The listing builds one solid part. Answer for the finished solid, in the listing's coordinates (mm). Face numbers are marked on the shaded views. A direction names the side the tool comes from. Give positions to 0.01 mm unless a question says otherwise; leave off trailing zeros. Write each loop counter-clockwise with the first axis right and the second up, starting at its lowest first coordinate (ties: lowest second). Pieces come first, ordered by that corner, then holes. Notation, with made-up numbers: (64, 22) - (109, 22) arc R14 cw to (109, 41) - close; hole circle Ø1 at (68.5, 16.5). An arc over 180 degrees is marked (long way). Answer as CSV lines item,"result". Start each with the question number.
(1) Find section D-D (x = 5.5). Write down the section's boundary in (y, z), then the cut area to 3 significant figures.
(2) Find section C-C (x = 26). Write down the section's boundary in (y, z).
(3) For a pull along Y with two mould halves and no side action, classify the marked faces 1, 2 and 3 as pulls with the +Y half, pulls with the -Y half, needs draft (parallel to the pull), parting line crosses it, or undercut.
(4) Find section B-B (z = 1). Write down the section's boundary in (x, y).
(5) Find section A-A (y = -3.5). Write down the section's boundary in (x, z), then the cut area to 4 significant figures.
(6) Each of these flat-tipped pins is pushed along its axis until it touches: pin 1 Ø5 at (x, y) = (31, 13) entering from +Z; pin 2 Ø7.5 at (y, z) = (12.5, 0) entering from +X; pin 3 Ø5 at (y, z) = (28.5, 0) entering from -X; pin 4 Ø1.6 at (x, z) = (6.5, 8.5) entering from -Y. Where does it stop, or does it pass through?
(7) Straight lines are drawn through the part: probe 1 along Y at (x, z) = (12.5, 0); probe 2 along X at (y, z) = (12.5, -6.5); probe 3 along Y at (x, z) = (7, 0). For each, find the intervals that lie inside material, in ascending order.
(8) For the marked faces 4, 5, 6, 7 and 8, determine the directions among +Z, -Z, +X, -X, +Y, -Y from which every point of the face is accessible in a straight line to the end or side of a thin tool.
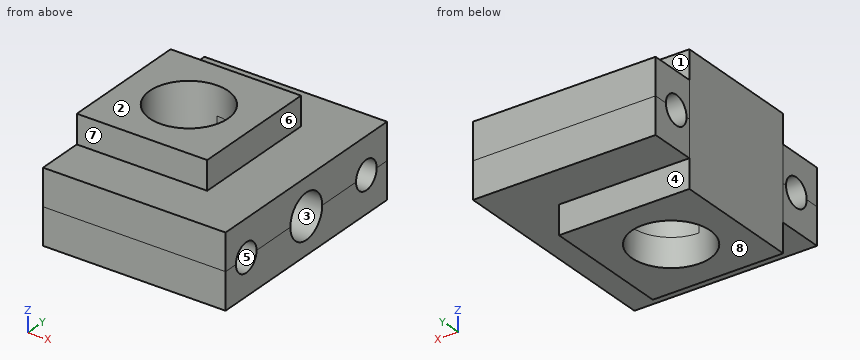
from build123d import *

# Parameters (mm, degrees)
F0_W          = 25
F0_H          = 25
F0_R          = 7.5
F1_DEPTH      = 12.5
F1_DEPTH_BACK = 12.5
F2_W          = 12.5
F2_H          = 9
F3_DEPTH      = 7
F3_DEPTH_BACK = 7
F6_DEPTH      = 10
F5_R          = 2.75
F7_DEPTH      = 35.1


with BuildPart() as f1:
    # F0 (on Top) → F1 (new body, two sides)
    with BuildSketch(Plane.XY) as f1_sk:
        with Locations((12.5, 12.5)):
            Rectangle(F0_W, F0_H)
        with Locations((12.5, 12.5)):
            Circle(F0_R, mode=Mode.SUBTRACT)
    extrude(amount=F1_DEPTH)
    extrude(f1_sk.sketch, amount=-F1_DEPTH_BACK)

    # F2 (on Top) → F3 (join, two sides)
    with BuildSketch(Plane.XY) as f3_sk:
        with BuildLine():
            Line((12.5, 34), (12.5, 25))
            Line((12.5, 25), (12.5, 20))
            ThreePointArc((12.5, 20), (17.803301, 17.803301), (20, 12.5))
            ThreePointArc((20, 12.5), (17.803301, 7.196699), (12.5, 5))
            Line((12.5, 5), (12.5, 0))
            Line((12.5, 0), (12.5, -9))
            Line((12.5, -9), (35, -9))
            Line((35, -9), (35, 34))
            Line((35, 34), (12.5, 34))
        make_face()
        with Locations((6.25, 29.5)):
            Rectangle(F2_W, F2_H)
        with Locations((6.25, -4.5)):
            Rectangle(F2_W, F2_H)
    extrude(amount=F3_DEPTH)
    extrude(f3_sk.sketch, amount=-F3_DEPTH_BACK)

    # F4 (on face) → F6 (cut)
    with BuildSketch(Plane.YZ.offset(35)):
        with BuildLine():
            ThreePointArc((8.25, 0), (12.5, -4.25), (16.75, 0))
            ThreePointArc((16.75, 0), (12.5, 4.25), (8.25, 0))
        make_face()
    extrude(amount=-F6_DEPTH, mode=Mode.SUBTRACT)

    # F5 (on face) → F7 (cut)
    with BuildSketch(Plane.YZ.offset(35)):
        with BuildLine():
            ThreePointArc((31.25, 0), (28.5, 2.75), (25.75, 0))
            ThreePointArc((25.75, 0), (28.5, -2.75), (31.25, 0))
        make_face()
        with Locations((-3.5, 0)):
            Circle(F5_R)
    extrude(amount=-F7_DEPTH, mode=Mode.SUBTRACT)


solid = f1.part
Result set:
1,outline,"(-9, -7) - (0, -7) - (0, -12.5) - (9.81, -12.5) - (9.81, 12.5) - (0, 12.5) - (0, 7) - (-9, 7) - close; (15.19, -12.5) - (25, -12.5) - (25, -7) - (34, -7) - (34, 7) - (25, 7) - (25, 12.5) - (15.19, 12.5) - close; hole circle Ø5.5 at (-3.5, 0); hole circle Ø5.5 at (28.5, 0)"
1,area,"695 mm^2"
2,outline,"(-9, -7) - (34, -7) - (34, 7) - (-9, 7) - close; hole circle Ø5.5 at (-3.5, 0); hole circle Ø8.5 at (12.5, 0); hole circle Ø5.5 at (28.5, 0)"
3,face 1,"pulls with the +Y half"
3,face 2,"needs draft"
3,face 3,"undercut"
4,outline,"(0, -9) - (35, -9) - (35, -6.06) - (0, -6.06) - close; (0, -0.94) - (35, -0.94) - (35, 8.37) - (25, 8.37) - (25, 16.63) - (35, 16.63) - (35, 25.94) - (0, 25.94) - close; (0, 31.06) - (35, 31.06) - (35, 34) - (0, 34) - close; hole circle Ø15 at (12.5, 12.5)"
5,outline,"(0, -7) - (35, -7) - (35, -2.75) - (0, -2.75) - close; (0, 2.75) - (35, 2.75) - (35, 7) - (0, 7) - close"
5,area,"297.5 mm^2"
6,pin 1,"z = 7"
6,pin 2,"x = 25"
6,pin 3,"through"
6,pin 4,"y = 0"
7,probe 1,"-9 to -6.25, -0.75 to 5, 20 to 25.75, 31.25 to 34"
7,probe 2,"0 to 5, 20 to 35"
7,probe 3,"-9 to -6.25, -0.75 to 7.4, 17.6 to 25.75, 31.25 to 34"
8,face 4,"-Z, +X, -X, +Y"
8,face 5,"+X, -X"
8,face 6,"+Z, +X, +Y, -Y"
8,face 7,"+Z, +X, -X, -Y"
8,face 8,"-Z, +X, -X, +Y, -Y"
